Can you work these out from the model? Positions are in its coordinate system, mm. Face numbers are marked on the shaded views. A direction names the side the tool comes from. Round coordinates to 2 decimals unless told otherwise and drop trailing zeros. Order: outer loops, then holes, each group sorted by start corner. A loop starts at its lowest first (then second) coordinate and runs counter-clockwise, first axis right, second up. Notation, with made-up numbers: (69.25, -33.5) -> (107.25, -33.5) arc R25 ccw to (107.25, -15.5) -> close; hole circle Ø5 at (-13, -19). An arc over 180 degrees is marked (long way). Use a Markdown table: item, result. Add a question column.
Q1. I'm going to push flat-ended pins straight in: pin 1 Ø1 at (x, z) = (-18, 23) entering from -Y; pin 2 Ø3 at (x, y) = (3.5, 3) entering from +Z; pin 3 Ø1.5 at (x, y) = (-31, 11) entering from -Z; pin 4 Ø6 at (x, y) = (13.5, 5) entering from +Z. Where does each tip first touch, or does it pass through?
Q2. If we section it at D-D on y = 8.5: List the corners of the cut face in (x, z) for me.
Q3. If we section it at A-A on x = 0: List the corners of the cut face in (y, z) for me.
Q4. For the marked faces 4 and 5, which set-ups out of +Z, -Z, +X, -X, +Y, -Y let a thin tool reach every point of the face, with its end or its side?
Q5. We'd pull the mould along X, two halves only. Please class the marked faces 1, 2 and 3: +X half, -X half, draft (parallel to the pull), parting line (faces both ways), or undercut.
Q6. If we section it at C-C on x = 30: List the corners of the cut face in (y, z) for me, plus the area to 3 significant figures.
Q7. I need wall thicknesses on line 1 along Z through (x, y) = (0, 1.65); line 2 along Y through (x, z) = (39.5, -17.5); line 3 along Y through (x, z) = (21.5, -12). Which ranges of each line are inside material? Lowest first, please. Write a range as [from, to].
Q8. If we section it at B-B on z = 0: List the corners of the cut face in (x, y) for me.
```python
from build123d import *

# Parameters (mm, degrees)
F_1_8_0_125_DIAMETER_HOLE1_D = 3.175


with BuildPart() as part:
    # Sketch1 → Revolve1 (revolve)
    with BuildSketch(Plane.XY):
        Polygon((-6.35, 0), (-6.35, 19.05), (-31.75, 19.05), (-31.75, 17.4625), (-44.45, 17.4625), (-44.45, 12.7), (-12.7, 12.7), (-12.7, 0), (-10.9855, 0), (-10.9855, 2.032), (-7.9375, 2.032), (-7.9375, 0), align=None)
    revolve(axis=Axis((0, 0, 0), (0, 1, 0)))

    # 1/8 (0.125) Diameter Hole1 (through all)
    with Locations(Plane(origin=(0, 17.4625, 0), x_dir=(1, 0, 0), z_dir=(0, 1, 0))):
        with Locations((-41.275, 0)):
            Hole(F_1_8_0_125_DIAMETER_HOLE1_D / 2)


solid = part.part
```
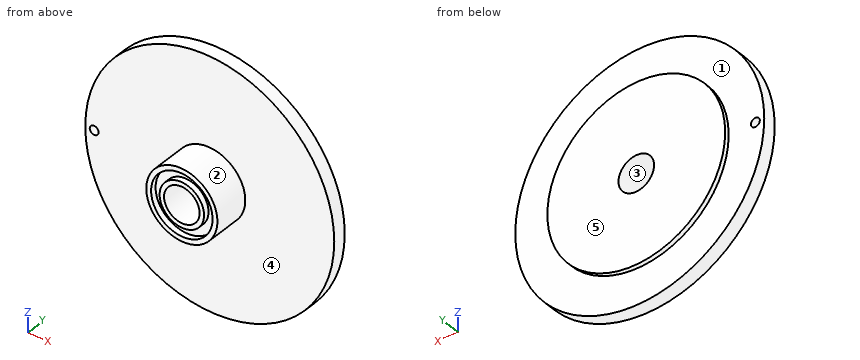
Answer below:
| question | item | result |
|---|---|---|
| 1 | pin 1 | y = 12.7 |
| 1 | pin 2 | z = 12.54 |
| 1 | pin 3 | through |
| 1 | pin 4 | z = 7.14 |
| 2 | outline | circle Ø25.4 at (0, 0); hole circle Ø12.7 at (0, 0) |
| 3 | outline | (0, -12.7) -> (12.7, -12.7) -> (12.7, -44.45) -> (17.46, -44.45) -> (17.46, -31.75) -> (19.05, -31.75) -> (19.05, -6.35) -> (0, -6.35) -> (0, -7.94) -> (2.03, -7.94) -> (2.03, -10.99) -> (0, -10.99) -> close; (0, 6.35) -> (19.05, 6.35) -> (19.05, 31.75) -> (17.46, 31.75) -> (17.46, 44.45) -> (12.7, 44.45) -> (12.7, 12.7) -> (0, 12.7) -> (0, 10.99) -> (2.03, 10.99) -> (2.03, 7.94) -> (0, 7.94) -> close |
| 4 | face 4 | -Y |
| 4 | face 5 | +Z, -Z, +X, -X, +Y |
| 5 | face 1 | draft |
| 5 | face 2 | parting line |
| 5 | face 3 | undercut |
| 6 | outline | (12.7, -32.8) -> (17.46, -32.8) -> (17.46, -10.4) -> (19.05, -10.4) -> (19.05, 10.4) -> (17.46, 10.4) -> (17.46, 32.8) -> (12.7, 32.8) -> close |
| 6 | area | 345 mm² |
| 7 | line 1 | [-12.7, -10.99], [-7.94, -6.35], [6.35, 7.94], [10.99, 12.7] |
| 7 | line 2 | [12.7, 17.46] |
| 7 | line 3 | [12.7, 19.05] |
| 8 | outline | (-44.45, 12.7) -> (-42.86, 12.7) -> (-42.86, 17.46) -> (-44.45, 17.46) -> close; (-39.69, 12.7) -> (-12.7, 12.7) -> (-12.7, 0) -> (-10.99, 0) -> (-10.99, 2.03) -> (-7.94, 2.03) -> (-7.94, 0) -> (-6.35, 0) -> (-6.35, 19.05) -> (-31.75, 19.05) -> (-31.75, 17.46) -> (-39.69, 17.46) -> close; (6.35, 0) -> (7.94, 0) -> (7.94, 2.03) -> (10.99, 2.03) -> (10.99, 0) -> (12.7, 0) -> (12.7, 12.7) -> (44.45, 12.7) -> (44.45, 17.46) -> (31.75, 17.46) -> (31.75, 19.05) -> (6.35, 19.05) -> close |
